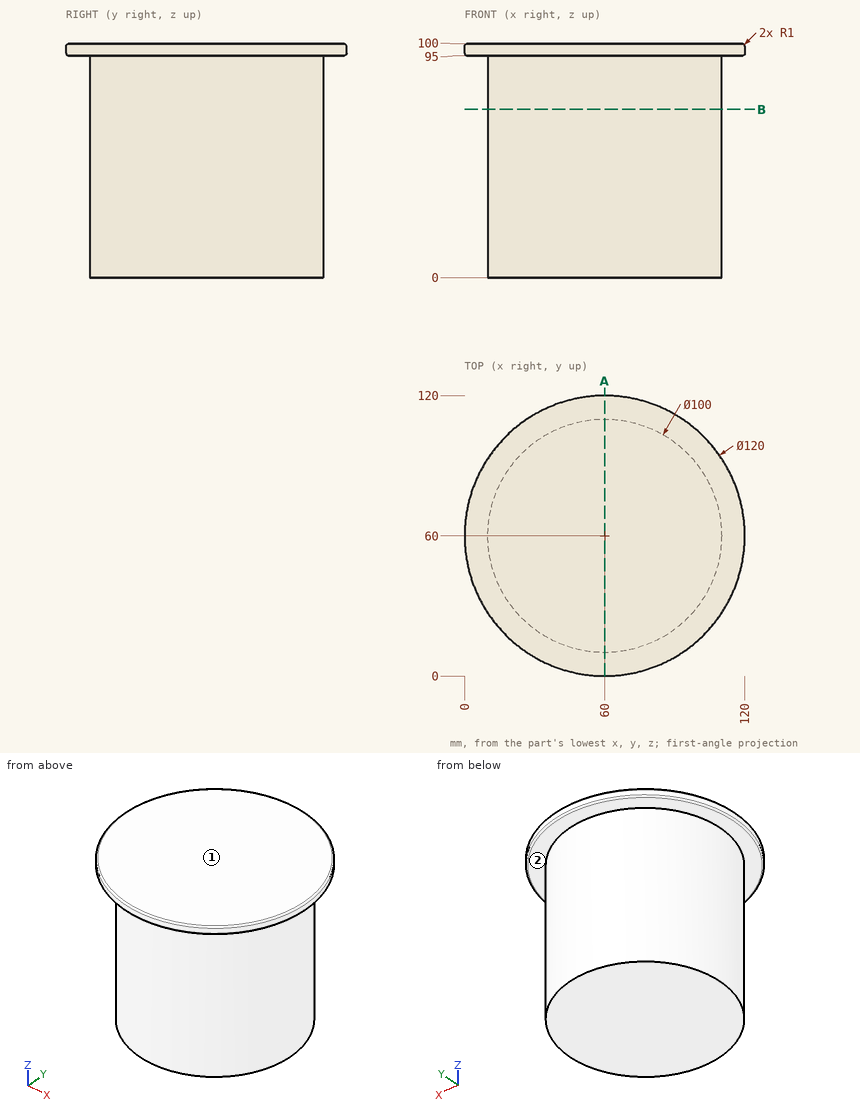
Source: three-view drawing plus pictorial views. Frame: mm from the lowest corner of the part. A direction names the side the tool comes from. Round coordinates to 2 decimals unless told otherwise and drop trailing zeros. Loops run counter-clockwise (first coordinate to the right, second up) from the corner with the lowest first, then second, coordinate; pieces in that order, holes last. Notation, with made-up numbers: (34, -30) - (85, -30) arc R10 cw to (85, -13) - close; hole circle Ø1 at (40, 51). An arc over 180 degrees is marked (long way). Write each question's results on one line, items separated by ' | '. Start each with the question number.
1) Cut plane A-A on x = 60. Return loops of the section in (y, z).
2) Line query: probe 1 along Z at (x, y) = (102, 92); probe 2 along Y at (x, z) = (104.5, 92); probe 3 along X at (y, z) = (39, 14.5). Output: solid intervals per line, ascending. Write a range as [from, to].
3) Cut plane B-B on z = 72. Return loops of the section in (x, y).
4) First-contact query: P1, Ø8, axis at y = 101, z = 28.5, coming from the +X side; P2, Ø12, axis at x = 71.5, z = 29, coming from the +Y side; P3, Ø8, axis at y = 91.5, z = 32.5, coming from the +X side. Flat tips, straight axial feed; report the tip coordinate or a pass-through.
5) Access query for the marked faces 1 and 2. Directions: +Z, -Z, +X, -X, +Y, -Y. A direction counts if a zero-diameter tool reaches every point of the face in a straight line with its end or side. Return the directions, or none.
Verdict:
1) outline: (0, 96) arc R1 ccw to (1, 95) - (10, 95) - (10, 0) - (110, 0) - (110, 95) - (119, 95) arc R1 ccw to (120, 96) - (120, 99) arc R1 ccw to (119, 100) - (1, 100) arc R1 ccw to (0, 99) - close
2) probe 1: z = [95, 100] | probe 2: y = [37.2, 82.8] | probe 3: x = [14.62, 105.38]
3) outline: circle Ø100 at (60, 60)
4) P1: stops at x = 93.63 | P2: stops at y = 109.7 | P3: stops at x = 101.76
5) face 1: +Z, +X, -X, +Y, -Y | face 2: -Z
